from build123d import *

# Parameters (mm, degrees)
SKETCH2_R           = 29.5
SKETCH2_R_2         = 4
BOSS_EXTRUDE2_DEPTH = 5


with BuildPart() as part:
    # Sketch2 → Boss-Extrude2 (new body)
    with BuildSketch(Plane.XY):
        Polygon((-40, 50), (-50, 40), (-50, -40), (-40, -50), (40, -50), (50, -40), (50, 40), (40, 50), align=None)
        Circle(SKETCH2_R, mode=Mode.SUBTRACT)
        with Locations((-40, 40)):
            Circle(SKETCH2_R_2, mode=Mode.SUBTRACT)
        with Locations((40, 40)):
            Circle(SKETCH2_R_2, mode=Mode.SUBTRACT)
        with Locations((40, -40)):
            Circle(SKETCH2_R_2, mode=Mode.SUBTRACT)
        with Locations((-40, -40)):
            Circle(SKETCH2_R_2, mode=Mode.SUBTRACT)
    extrude(amount=BOSS_EXTRUDE2_DEPTH)


solid = part.part
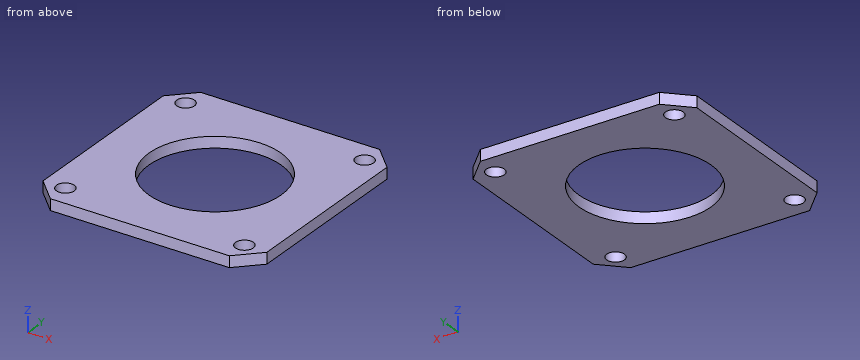
Design review of the part built by this model. Coordinates are the model's own, in mm. Coordinates: 2 decimals unless noted, no trailing zeros. Order: outer loops, then holes, each group sorted by start corner. A loop starts at its lowest first (then second) coordinate and runs counter-clockwise, first axis right, second up.
Item 1: Take a section at C-C, the plane z = 2.35. Write out the cut boundary in (x, y), then the cut area to 3 significant figures.
Item 2: Take a section at D-D, the plane x = 42. Write out the cut boundary in (y, z), then the cut area to 3 significant figures.
Item 3: Take a section at A-A, the plane x = 0. Write out the cut boundary in (y, z).
Item 4: For line 1 (Y direction, x = 40, z = 3); line 2 (X direction, y = 38, z = 4.75); line 3 (Y direction, x = 0, z = 3.45), list the stretches that pass through material, from the lowest coordinate up.
Item 5: For pin 1 Ø8 at (x, y) = (-4, 25.5) entering from -Z, flat-tipped, find the tip position at first contact; note if it passes through.
The answers:
1. outline: (-50, -40) - (-40, -50) - (40, -50) - (50, -40) - (50, 40) - (40, 50) - (-40, 50) - (-50, 40) - close; hole circle Ø8 at (-40, -40); hole circle Ø8 at (-40, 40); hole circle Ø59 at (0, 0); hole circle Ø8 at (40, -40); hole circle Ø8 at (40, 40)
1. area: 6,860 mm2
2. outline: (-48, 0) - (-43.46, 0) - (-43.46, 5) - (-48, 5) - close; (-36.54, 0) - (36.54, 0) - (36.54, 5) - (-36.54, 5) - close; (43.46, 0) - (48, 0) - (48, 5) - (43.46, 5) - close
2. area: 411 mm2
3. outline: (-50, 0) - (-29.5, 0) - (-29.5, 5) - (-50, 5) - close; (29.5, 0) - (50, 0) - (50, 5) - (29.5, 5) - close
4. line 1: y = -50 to -44, -36 to 36, 44 to 50
4. line 2: x = -50 to -43.46, -36.54 to 36.54, 43.46 to 50
4. line 3: y = -50 to -29.5, 29.5 to 50
5. pin 1: stops at z = 0
